Read the model definition and answer for the solid it produces. Units are mm, in the model's axes. Give positions to 0.01 mm unless a question says otherwise; leave off trailing zeros. Order: outer loops, then holes, each group sorted by start corner. A loop starts at its lowest first (then second) coordinate and runs counter-clockwise, first axis right, second up. Notation, with made-up numbers: (-17, 47.5) - (-6, 47.5) arc R6 cw to (-6, 53.5) - close; hole circle Ø4 at (-11.75, 6.25). An arc over 180 degrees is marked (long way). Use a Markdown table: item, result. Add a question column.
1. A cutting plane is placed at C-C on x = -45. Determine the outline of the cut face in (y, z).
2. A cutting plane is placed at A-A on x = -70. Determine the outline of the cut face in (y, z), and give its area (4 significant figures).
3. A cutting plane is placed at B-B on z = -170. Determine the outline of the cut face in (x, y), and give its area (4 significant figures).
4. A flat-ended cylindrical pin translates along its axis: P1, Ø4.5, axis at x = -45, z = -130, coming from the +Y side. Find the tip coordinate at first contact, or state that the pin passes through.
5. Consider L1, parallel to X at y = 2.5, z = -165; L2, parallel to Z at x = -45, y = 2.95; L3, parallel to Z at x = -10, y = 1.9. Determine where each line is inside the solid, lowest interval first.
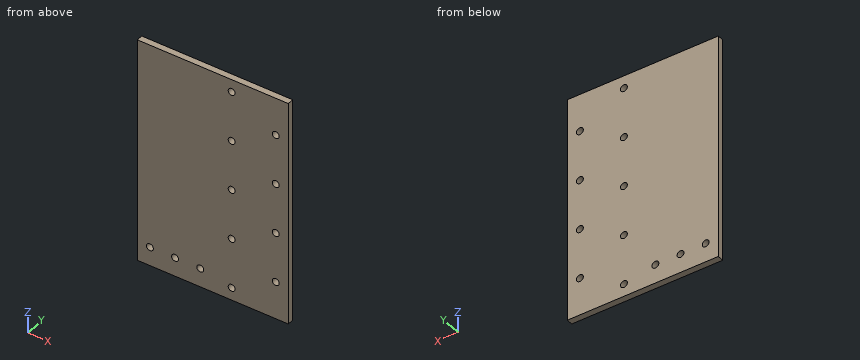
Autodesk Inventor part; units mm, degrees
ref_plane "YZ Plane" through (0, 0, 0) normal (1, 0, 0) x (0, 1, 0)
ref_plane "XZ Plane" through (0, 0, 0) normal (0, 1, 0) x (-1, 0, 0)
ref_plane "XY Plane" through (0, 0, 0) normal (0, 0, 1) x (1, 0, 0)
sketch "Sketch1" plane through (0, 0, 0) normal (0, 1, 0) x (-1, 0, 0)
  line L0 (0, 0) -> (120, 0)
  line L1 (120, 0) -> (120, -180)
  line L2 (120, -180) -> (0, -180)
  line L3 (0, -180) -> (0, 0)
  dimension "d0" = 120
  dimension "d1" = 180
extrude "Extrusion1" add sketch "Sketch1" along normal blind 5
sketch "Sketch2" plane through (0, 5, 0) normal (0, 1, 0) x (1, 0, 0)
  circle A0 centre (-45, 10) radius 2.75
  line L0 (-120, 0) -> (0, 0)
  line L1 (0, 0) -> (0, 180)
  circle A1 centre (-45, 50) radius 2.75
  circle A2 centre (-45, 90) radius 2.75
  circle A3 centre (-45, 130) radius 2.75
  circle A4 centre (-45, 170) radius 2.75
  circle A5 centre (-10, 30) radius 2.75
  circle A6 centre (-10, 70) radius 2.75
  circle A7 centre (-10, 110) radius 2.75
  circle A8 centre (-10, 150) radius 2.75
  dimension "d4" = 5.5
  dimension "d5" = 10
  dimension "d8" = 40
  dimension "d13" = 45
  dimension "d14" = 5.5
  dimension "d15" = 10
  dimension "d16" = 180
  dimension "d17" = 30
  dimension "d20" = 40
extrude "Extrusion2" cut sketch "Sketch2" against normal blind 5
sketch "Sketch3" plane through (0, 5, 0) normal (0, 1, 0) x (1, 0, 0)
  circle A0 centre (-110, 165) radius 2.75
  line L0 (0, 180) -> (-120, 180)
  circle A1 centre (-90, 165) radius 2.75
  circle A2 centre (-70, 165) radius 2.75
  line L1 (-120, 180) -> (-120, 0)
  point P0 (0, 0)
  dimension "d27" = 5.5
  dimension "d28" = 15
  dimension "d31" = 20
  dimension "d38" = 10
extrude "Extrusion3" cut sketch "Sketch3" against normal blind 5
properties part number "GanrtyPlatev2"
Output values:
| question | item | result |
|---|---|---|
| 1 | outline | (0, -180) - (5, -180) - (5, -172.75) - (0, -172.75) - close; (0, -167.25) - (5, -167.25) - (5, -132.75) - (0, -132.75) - close; (0, -127.25) - (5, -127.25) - (5, -92.75) - (0, -92.75) - close; (0, -87.25) - (5, -87.25) - (5, -52.75) - (0, -52.75) - close; (0, -47.25) - (5, -47.25) - (5, -12.75) - (0, -12.75) - close; (0, -7.25) - (5, -7.25) - (5, 0) - (0, 0) - close |
| 2 | outline | (0, -180) - (5, -180) - (5, -167.75) - (0, -167.75) - close; (0, -162.25) - (5, -162.25) - (5, 0) - (0, 0) - close |
| 2 | area | 872.5 mm² |
| 3 | outline | (-120, 0) - (-47.75, 0) - (-47.75, 5) - (-120, 5) - close; (-42.25, 0) - (0, 0) - (0, 5) - (-42.25, 5) - close |
| 3 | area | 572.5 mm² |
| 4 | P1 | through |
| 5 | L1 | -120 to -112.75, -107.25 to -92.75, -87.25 to -72.75, -67.25 to 0 |
| 5 | L2 | -180 to -172.75, -167.25 to -132.75, -127.25 to -92.75, -87.25 to -52.75, -47.25 to -12.75, -7.25 to 0 |
| 5 | L3 | -180 to -152.75, -147.25 to -112.75, -107.25 to -72.75, -67.25 to -32.75, -27.25 to 0 |
